Can you work these out from the model? Positions are in its coordinate system, mm. A direction names the side the tool comes from. Coordinates: 2 decimals unless noted, no trailing zeros. Order: outer loops, then holes, each group sorted by start corner. A loop starts at its lowest first (then second) coordinate and runs counter-clockwise, first axis right, second up. Notation, with made-up numbers: (-7, 30) -> (44, 30) arc R15 cw to (44, 55) -> close; hole circle Ø3 at (61, -37.75). An arc over 180 degrees is marked (long way). Answer in a Markdown table with one row per item. Add a question column.
1. Imagine slicing it at C-C on y = 15. Write out the boundary of the cut face in (x, z).
2. Imagine slicing it at B-B on z = 14.75. Write out the boundary of the cut face in (x, y).
3. Imagine slicing it at D-D on z = 8.75. Write out the boundary of the cut face in (x, y), plus the area to 3 significant figures.
4. If I drill on line 1 along Y through (x, z) = (27, 3.25); line 2 along X through (y, z) = (17.5, 2.75); line 3 along X through (y, z) = (26, 11), over which ranges is the centre line in solid material (lowest first)? Write a range as [from, to].
5. On a 3-axis mill with a long thin cutter (end or side, diameter ignored), from which of +Z, -Z, +X, -X, +Y, -Y can I reach the whole of each face in a straight line? I mean faces 1 (the face through (28, -2, 17.264)), 2 (the face through (63, 22, 7)), 3 (the face through (0, 17, 2)). Say none if no direction works.
6. Imagine slicing it at A-A on z = 2.25. Write out the boundary of the cut face in (x, y), plus the area to 3 significant figures.
7. We'd pull the mould along Z, two halves only. Please class faces 4 (the face through (31, -1, 9)), 5 (the face through (-2, 12, 7)), 6 (the face through (30, 17, 0)), 7 (the face through (30, 17, 1.5)): pulls with the +Z half, pulls with the -Z half, needs draft (parallel to the pull), parting line crosses it, or undercut.
8. Will this pin go through, and if not, where does the flat tip stop? pin 1 (5 mm diameter, centred on x = 47, y = 20.5, fed in from +Z).
Autodesk Fusion 360 part; units mm, degrees
sketch "Spodek" plane through (0, 0, 0) normal (0, 0, 1) x (1, 0, 0)
  line L0 (0, 0) -> (61, 0)
  line L1 (61, 0) -> (61, 34)
  line L2 (61, 34) -> (0, 34)
  line L3 (0, 34) -> (0, 0)
  line L4 (-1, 35) -> (62, 35)
  line L5 (62, 35) -> (62, -1)
  line L6 (62, -1) -> (-1, -1)
  line L7 (-1, -1) -> (-1, 35)
  line L8 (-2.7, -2.7) -> (-2.7, 36.7) construction
  line L9 (63.7, 36.7) -> (-2.7, 36.7) construction
  line L10 (63.7, -2.7) -> (63.7, 36.7) construction
  line L11 (63.7, -2.7) -> (-2.7, -2.7) construction
  line L12 (-2.7, -2.7) -> (63.7, -2.7)
  line L13 (63.7, -2.7) -> (63.7, 36.7)
  line L14 (63.7, 36.7) -> (-2.7, 36.7)
  line L15 (-2.7, 36.7) -> (-2.7, -2.7)
  dimension "d1" = 61
  dimension "d2" = 34
  dimension "d3" = 63
  dimension "d4" = 36
  dimension "d5" = 1.7
  dimension "d6" = 1.7
  dimension "d7" = 1.7
  dimension "d8" = 1.7
sketch "TotoNevim" plane through (0, 0, 0) normal (0, 0, 1) x (1, 0, 0)
extrude "Extrude1" add sketch "Spodek" along normal blind 12 contours L12 L13 L14 L15
extrude "Extrude2" add sketch "Spodek" along normal blind 1.5 contours L0 L1 L2 L3 | L4 L5 L6 L7
sketch "Sketch3" plane through (0, 0, 1.5) normal (0, 0, 1) x (-1, 0, 0)
  line L0 (1, 1) -> (-62, 1)
  line L1 (-62, 1) -> (-62, -35)
  line L2 (-62, -35) -> (1, -35)
  line L3 (1, -35) -> (1, 1)
  line L4 (-59.78, -32.78) -> (-1.22, -32.78)
  line L5 (-1.22, -32.78) -> (-1.22, -1.22)
  line L6 (-1.22, -1.22) -> (-59.78, -1.22)
  line L7 (-59.78, -1.22) -> (-59.78, -32.78)
  line L8 (-61, 0) -> (-61, -34)
  line L9 (0, 0) -> (-61, 0)
  line L10 (0, -34) -> (0, 0)
  line L11 (-61, -34) -> (0, -34)
  dimension "d13" = 1.22
  dimension "d14" = 1.22
  dimension "d15" = 1.22
  dimension "d16" = 1.22
extrude "Extrude3" add sketch "Sketch3" along normal blind 1.8 contours L8 L9 L10 L11
extrude "Extrude4" add 1 faces at (20, -2.1333, 12) along direction (0, 0, 1) blind 5.243
extrude "Extrude5" add 1 faces at (20, -2.1333, 17.243) along direction (0, 0, 1) blind 0.021
sketch "Prurez1" plane through (-2.7, 0, 0) normal (-1, 0, 0) x (0, -1, 0)
  line L0 (-36.7, 0) -> (2.7, 0)
  line L1 (2.7, 0) -> (2.7, 17.264)
  line L2 (2.7, 17.264) -> (-36.7, 17.264)
  line L3 (-36.7, 17.264) -> (-36.7, 0)
  line L4 (-12, 3.3) -> (-12, 11) construction
  line L5 (0, 1.5) -> (0, 3.3) construction
  line L6 (-22, 11) -> (-22, 3.3) construction
  line L7 (-34, 3.3) -> (-34, 11) construction
  line L8 (-35, 1.5) -> (-35, 17.264) construction
  line L9 (-22, 11) -> (-12, 11) construction
  line L10 (-12, 11) -> (-12, 3.3) construction
  line L11 (-12, 3.3) -> (-22, 3.3) construction
  line L12 (-22, 3.3) -> (-22, 11) construction
  line L13 (-22, 11) -> (-12, 11)
  line L14 (-12, 11) -> (-12, 3.3)
  line L15 (-12, 3.3) -> (-22, 3.3)
  line L16 (-22, 3.3) -> (-22, 11)
  dimension "d23" = 7.7
  dimension "d24" = 12
  dimension "d25" = 12
  dimension "d26" = 1
extrude "Extrude6" cut sketch "Prurez1" against normal up to surface (66.4 mm away) contours L13 L14 L15 L16
equation "d19 = 14 mm - 8.757 mm"
equation "d21 = 14 mm - 13.979 mm"
Answers follow:
| question | item | result |
|---|---|---|
| 1 | outline | (-2.7, 0) -> (63.7, 0) -> (63.7, 3.3) -> (62, 3.3) -> (62, 1.5) -> (61, 1.5) -> (61, 3.3) -> (59.78, 3.3) -> (59.78, 1.5) -> (1.22, 1.5) -> (1.22, 3.3) -> (0, 3.3) -> (0, 1.5) -> (-1, 1.5) -> (-1, 3.3) -> (-2.7, 3.3) -> close; (-2.7, 11) -> (-1, 11) -> (-1, 17.26) -> (-2.7, 17.26) -> close; (62, 11) -> (63.7, 11) -> (63.7, 17.26) -> (62, 17.26) -> close |
| 2 | outline | (-2.7, -2.7) -> (63.7, -2.7) -> (63.7, 36.7) -> (-2.7, 36.7) -> close; hole (-1, -1) -> (62, -1) -> (62, 35) -> (-1, 35) -> close |
| 3 | outline | (-2.7, -2.7) -> (63.7, -2.7) -> (63.7, 12) -> (62, 12) -> (62, -1) -> (-1, -1) -> (-1, 12) -> (-2.7, 12) -> close; (-2.7, 22) -> (-1, 22) -> (-1, 35) -> (62, 35) -> (62, 22) -> (63.7, 22) -> (63.7, 36.7) -> (-2.7, 36.7) -> close |
| 3 | area | 314 mm² |
| 4 | line 1 | y = [-2.7, -1], [0, 1.22], [32.78, 34], [35, 36.7] |
| 4 | line 2 | x = [-2.7, -1], [0, 1.22], [59.78, 61], [62, 63.7] |
| 4 | line 3 | x = [-2.7, -1], [62, 63.7] |
| 5 | face 1 | +Z, +X, -X, +Y, -Y |
| 5 | face 2 | +X, -X |
| 5 | face 3 | +Z |
| 6 | outline | (-2.7, -2.7) -> (63.7, -2.7) -> (63.7, 36.7) -> (-2.7, 36.7) -> close; (0, 0) -> (61, 0) -> (61, 34) -> (0, 34) -> close; hole (-1, -1) -> (62, -1) -> (62, 35) -> (-1, 35) -> close; hole (1.22, 1.22) -> (59.78, 1.22) -> (59.78, 32.78) -> (1.22, 32.78) -> close |
| 6 | area | 574 mm² |
| 7 | face 4 | needs draft |
| 7 | face 5 | undercut |
| 7 | face 6 | pulls with the -Z half |
| 7 | face 7 | pulls with the +Z half |
| 8 | pin 1 | stops at z = 1.5 |
